from build123d import *
from build123d import SkipClean  # not in build123d's __all__

# Parameters (mm, degrees)
F2_R      = 21
F3_DEPTH  = 3
F4_R      = 10
F5_DEPTH  = 2
F6_R      = 5
F7_DEPTH  = 25
F8_R      = 5
F9_DEPTH  = 3
F10_R     = 5.5
F11_DEPTH = 1
F12_DEPTH = 1
F13_R     = 5.5
F14_DEPTH = 1
F15_R     = 5
F16_DEPTH = 1
F17_DEPTH = 2


# Not quite as in the source:
# - the program builds the solid bodies; features that only make, move or delete a surface that nothing else refers to are left out


with BuildPart() as f3:
    # F2 (on Front) → F3 (new body)
    with BuildSketch(Plane.XZ):
        Circle(F2_R)
    extrude(amount=F3_DEPTH)

    # F4 (on Front) → F5 (join)
    with BuildSketch(Plane.XZ):
        Circle(F4_R)
    extrude(amount=-F5_DEPTH)

    # F6 (on face) → F7 (cut)
    with BuildSketch(Plane(origin=(0, 2, 0), x_dir=(-1, 0, 0), z_dir=(0, 1, 0))):
        Circle(F6_R)
    extrude(amount=-F7_DEPTH, mode=Mode.SUBTRACT)

    # F8 (on face) → F9 (join)
    with BuildSketch(Plane.XZ.offset(3)):
        with Locations((6.0798030726, 20.1006466214)):
            Circle(F8_R)
        with BuildLine():
            ThreePointArc((10.6593068139, 18.093622585), (6.0798030726, 20.1006466214), (1.1556392931, 20.968178219))
            ThreePointArc((1.1556392931, 20.968178219), (4.6322309124, 15.3147783782), (10.6593068139, 18.093622585))
        make_face()
    extrude(amount=-F9_DEPTH)

    # F10 (on face) → F11 (join)
    with BuildSketch(Plane.XZ.offset(3)):
        with BuildLine():
            ThreePointArc((10.6593068139, 18.093622585), (7.5273752327, 24.8865148646), (1.1556392931, 20.968178219))
            ThreePointArc((1.1556392931, 20.968178219), (-6.0798030726, -20.1006466214), (10.6593068139, 18.093622585))
        make_face()
        Circle(F10_R, mode=Mode.SUBTRACT)
    with SkipClean():  # cleaning this boolean's faces spoils the solid; the shape is the same uncleaned
        extrude(amount=F11_DEPTH)

    # F12 (add): a face of the model
    f12_faces = [f3.faces().sort_by_distance(p)[0] for p in [
        (-5.3444365081, -3, 0),
    ]]
    with SkipClean():  # cleaning this boolean's faces spoils the solid; the shape is the same uncleaned
        extrude(f12_faces, amount=F12_DEPTH)

    # F13 (on face) → F14 (join)
    with BuildSketch(Plane.XZ.offset(4)):
        with BuildLine():
            ThreePointArc((10.6593068139, 18.093622585), (7.5273752327, 24.8865148646), (1.1556392931, 20.968178219))
            ThreePointArc((1.1556392931, 20.968178219), (-6.0798030726, -20.1006466214), (10.6593068139, 18.093622585))
        make_face()
        Circle(F13_R, mode=Mode.SUBTRACT)
    extrude(amount=F14_DEPTH)

    # F15 (on face) → F16 (cut)
    with BuildSketch(Plane.XZ.offset(5)):
        Circle(F15_R)
    extrude(amount=-F16_DEPTH, mode=Mode.SUBTRACT)

    # F17 (add): a face of the model
    f17_faces = [f3.faces().sort_by_distance(p)[0] for p in [
        (-5.3444365081, -4, 0),
    ]]
    extrude(f17_faces, amount=F17_DEPTH)


solid = f3.part
Design review of the part built by this model. Coordinates are the model's own, in mm. A direction names the side the tool comes from. Round coordinates to 2 decimals unless told otherwise and drop trailing zeros. Loops run counter-clockwise (first coordinate to the right, second up) from the corner with the lowest first, then second, coordinate; pieces in that order, holes last. Notation, with made-up numbers: (38.5, 39) -> (49.5, 39) arc R21 cw to (49.5, 54) -> close; hole circle Ø11 at (33.25, 86.25). An arc over 180 degrees is marked (long way). Use one line per item in the form item = value. Start each with the question number.
Q1. We need section B-B on z = 0. Give the boundary of the cut face in (x, y).
Q2. We need section C-C on y = 1. Give the boundary of the cut face in (x, z).
Q3. We need section A-A on x = 0. Give the boundary of the cut face in (y, z), then the cut area to 3 significant figures.
Q4. Wall thickness on line 1 along X through (y, z) = (-4.6, 0); line 2 along Z through (x, y) = (0, -5.15): over which ranges is each line inside the solid? List them lowest first. Write a range as [from, to].
Q5. We need section D-D on z = 15.5. Give the boundary of the cut face in (x, y), then the cut area to 3 significant figures.
Q6. Machinability: for faces 1 (the face through (-1.19, -5.49, -5.37)), 2 (the face through (1.6, -6, -4.9)), 3 (the face through (-10, 0, -3)), which of the approach directions +Z, -Z, +X, -X, +Y, -Y give a long, thin tool a straight path to every point of the face, cutting with its end or side? Answer none if there is none.
Q7. For pin 1 Ø10 at (x, z) = (-10, -3.5) entering from -Y; pin 2 Ø3 at (x, z) = (2.5, -11.5) entering from +Y, all flat-tipped, find the tip position at first contact; note any pin that passes through.
Calculated:
q1.outline = (-21, -5) -> (-5.5, -5) -> (-5.5, -6) -> (-5, -6) -> (-5, 2) -> (-10, 2) -> (-10, 0) -> (-21, 0) -> close; (5, -6) -> (5.5, -6) -> (5.5, -5) -> (21, -5) -> (21, 0) -> (10, 0) -> (10, 2) -> (5, 2) -> close
q2.outline = circle Ø20 at (0, 0); hole circle Ø10 at (0, 0)
q3.outline = (-6, -5.5) -> (-5, -5.5) -> (-5, -21) -> (0, -21) -> (0, -10) -> (2, -10) -> (2, -5) -> (-6, -5) -> close; (-6, 5) -> (2, 5) -> (2, 10) -> (0, 10) -> (0, 21) -> (-5, 21) -> (-5, 5.5) -> (-6, 5.5) -> close
q3.area = 181 mm²
q4.line_1 = [-21, -5], [5, 21]
q4.line_2 = [-5.5, -5], [5, 5.5]
q5.outline = (-14.17, -5) -> (14.17, -5) -> (14.17, 0) -> (-14.17, 0) -> close
q5.area = 142 mm²
q6.face_1 = -Y
q6.face_2 = +Z, -Z, +X, -X, -Y
q6.face_3 = +Y
q7.pin_1 = -5
q7.pin_2 = 0
